For this review, take the finished solid that the model builds, in its own axes (mm). Face numbers are marked on the shaded views. Coordinates: 2 decimals unless noted, no trailing zeros. Write each loop counter-clockwise with the first axis right and the second up, starting at its lowest first coordinate (ties: lowest second). Pieces come first, ordered by that corner, then holes. Notation, with made-up numbers: M 21,37.25 L 49,37.25 A10 cw 49,56.25 Z; hole C 87,52 d7. An arc over 180 degrees is marked long. One line per question, with ' | ' between items.
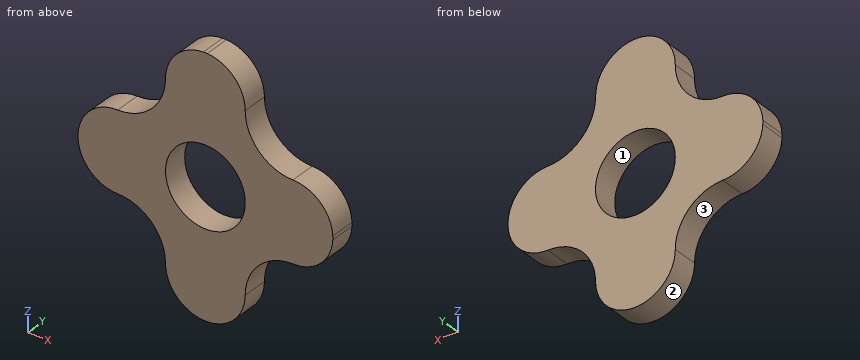
from build123d import *

# Parameters (mm, degrees)
F0_R      = 35.56
F1_DEPTH  = 7.1882
F2_R      = 11.1379
F3_DEPTH  = 7.62
F7_DEPTH  = 7.1882
F9_DEPTH  = 7.1882
F11_DEPTH = 7.1882
F13_DEPTH = 7.1882
F15_DEPTH = 25.4


# Not quite as in the source:
# - a feature of the source that left no trace in its solid (it failed there, or was rolled back) is left out


with BuildPart() as f1:
    # F0 (on Front) → F1 (new body)
    with BuildSketch(Plane.XZ):
        Circle(F0_R)
    extrude(amount=F1_DEPTH)

    # F2 (on face) → F3 (cut)
    with BuildSketch(Plane(origin=(0, 0, 0), x_dir=(-1, 0, 0), z_dir=(0, 1, 0))):
        Circle(F2_R)
    extrude(amount=-F3_DEPTH, mode=Mode.SUBTRACT)

    # F6 (on face) → F7 (join)
    with BuildSketch(Plane.XZ.offset(7.1882)):
        with BuildLine():
            Line((35.56, 11.1379), (33.7707089589, 11.1379))
            ThreePointArc((33.7707089589, 11.1379), (35.1098277593, 5.6403541298), (35.56, 0))
            Line((35.56, 0), (35.56, 11.1379))
        make_face()
        with BuildLine():
            Line((35.56, -11.1125), (35.56, 0))
            ThreePointArc((35.56, 0), (35.1119461572, -5.6271517709), (33.7790755313, -11.1125))
            Line((33.7790755313, -11.1125), (35.56, -11.1125))
        make_face()
    extrude(amount=-F7_DEPTH)

    # F8 (on face) → F9 (join)
    with BuildSketch(Plane.XZ.offset(7.1882)):
        with BuildLine():
            Line((-11.1379, 35.56), (-11.1379, 33.7707089589))
            ThreePointArc((-11.1379, 33.7707089589), (-5.6403540801, 35.1098277673), (1.006e-07, 35.56))
            Line((1.006e-07, 35.56), (-11.1379, 35.56))
        make_face()
        with BuildLine():
            Line((11.1125, 35.56), (1.006e-07, 35.56))
            ThreePointArc((1.006e-07, 35.56), (5.6271518206, 35.1119461492), (11.1125, 33.7790755313))
            Line((11.1125, 33.7790755313), (11.1125, 35.56))
        make_face()
    extrude(amount=-F9_DEPTH)

    # F10 (on face) → F11 (join)
    with BuildSketch(Plane.XZ.offset(7.1882)):
        with BuildLine():
            ThreePointArc((-35.56, 0), (-35.1119461572, 5.627151771), (-33.7790755313, 11.1125))
            Line((-33.7790755313, 11.1125), (-35.56, 11.1125))
            Line((-35.56, 11.1125), (-35.56, 0))
        make_face()
        with BuildLine():
            Line((-35.56, -11.1379), (-33.7707089589, -11.1379))
            ThreePointArc((-33.7707089589, -11.1379), (-35.1098277593, -5.6403541298), (-35.56, 0))
            Line((-35.56, 0), (-35.56, -11.1379))
        make_face()
    extrude(amount=-F11_DEPTH)

    # F12 (on face) → F13 (join)
    with BuildSketch(Plane.XZ.offset(7.1882)):
        with BuildLine():
            ThreePointArc((0, -35.56), (-5.6403541298, -35.1098277593), (-11.1379, -33.7707089589))
            Line((-11.1379, -33.7707089589), (-11.1379, -35.56))
            Line((-11.1379, -35.56), (0, -35.56))
        make_face()
        with BuildLine():
            Line((11.1125, -35.56), (11.1125, -33.7790755313))
            ThreePointArc((11.1125, -33.7790755313), (5.6271517709, -35.1119461572), (0, -35.56))
            Line((0, -35.56), (11.1125, -35.56))
        make_face()
    extrude(amount=-F13_DEPTH)

    # F14 (on face) → F15 (cut)
    with BuildSketch(Plane.XZ.offset(7.1882)):
        with BuildLine():
            ThreePointArc((-11.1379, 24.4221), (-8.0739891454, 32.1147190965), (-0.5444488019, 35.56))
            Line((-0.5444488019, 35.56), (-11.1379, 35.56))
            Line((-11.1379, 35.56), (-11.1379, 33.7707089589))
            ThreePointArc((-11.1379, 33.7707089589), (-25.1541702512, 25.1352604716), (-33.7790755313, 11.1125))
            Line((-33.7790755313, 11.1125), (-35.56, 11.1125))
            Line((-35.56, 11.1125), (-35.56, 0.5190198064))
            ThreePointArc((-35.56, 0.5190198064), (-32.1239164631, 8.03980237), (-24.4475, 11.1125))
            ThreePointArc((-24.4475, 11.1125), (-15.0361915851, 15.0107915851), (-11.1379, 24.4221))
        make_face()
        with BuildLine():
            Line((-0.5444488019, 35.56), (0.5190198064, 35.56))
            ThreePointArc((0.5190198064, 35.56), (-0.0127144977, 35.5727144977), (-0.5444488019, 35.56))
        make_face()
        with BuildLine():
            ThreePointArc((0.5190198064, 35.56), (8.03980237, 32.1239164631), (11.1125, 24.4475))
            ThreePointArc((11.1125, 24.4475), (15.0107915851, 15.0361915851), (24.4221, 11.1379))
            ThreePointArc((24.4221, 11.1379), (32.1147190965, 8.0739891454), (35.56, 0.5444488019))
            Line((35.56, 0.5444488019), (35.56, 11.1379))
            Line((35.56, 11.1379), (33.7707089589, 11.1379))
            ThreePointArc((33.7707089589, 11.1379), (25.1352604716, 25.1541702512), (11.1125, 33.7790755313))
            Line((11.1125, 33.7790755313), (11.1125, 35.56))
            Line((11.1125, 35.56), (0.5190198064, 35.56))
        make_face()
        with BuildLine():
            ThreePointArc((35.56, -0.5190198064), (35.5727144977, 0.0127144977), (35.56, 0.5444488019))
            Line((35.56, 0.5444488019), (35.56, -0.5190198064))
        make_face()
        with BuildLine():
            Line((35.56, -11.1125), (35.56, -0.5190198064))
            ThreePointArc((35.56, -0.5190198064), (32.1239164631, -8.03980237), (24.4475, -11.1125))
            ThreePointArc((24.4475, -11.1125), (15.0182310729, -15.0182310729), (11.1125, -24.4475))
            ThreePointArc((11.1125, -24.4475), (-0.0253855106, -35.5473072489), (-11.1379, -24.4221))
            ThreePointArc((-11.1379, -24.4221), (-15.0287520974, -15.0287520974), (-24.4221, -11.1379))
            ThreePointArc((-24.4221, -11.1379), (-32.1147190965, -8.0739891454), (-35.56, -0.5444488019))
            Line((-35.56, -0.5444488019), (-35.56, -11.1379))
            Line((-35.56, -11.1379), (-33.7707089589, -11.1379))
            ThreePointArc((-33.7707089589, -11.1379), (-25.144717139, -25.144717139), (-11.1379, -33.7707089589))
            Line((-11.1379, -33.7707089589), (-11.1379, -35.56))
            Line((-11.1379, -35.56), (11.1125, -35.56))
            Line((11.1125, -35.56), (11.1125, -33.7790755313))
            ThreePointArc((11.1125, -33.7790755313), (25.144717139, -25.144717139), (33.7790755313, -11.1125))
            Line((33.7790755313, -11.1125), (35.56, -11.1125))
        make_face()
        with BuildLine():
            Line((-35.56, -0.5444488019), (-35.56, 0.5190198064))
            ThreePointArc((-35.56, 0.5190198064), (-35.5727144977, -0.0127144977), (-35.56, -0.5444488019))
        make_face()
    extrude(amount=-F15_DEPTH, mode=Mode.SUBTRACT)


solid = f1.part
1. Take a section at D-D on z = -29. State the section outline as (x, y) points, plus the area to 3 significant figures.
Computed values:
outline: M -10.15,-7.19 L 10.13,-7.19 L 10.13,0 L -10.15,0 Z | area: 146 mm2
2. Clearance check with flat-ended pins moving along their axes: P1, Ø1.5, axis at x = 24.5, y = -6.5, coming from the +Z side; P2, Ø20, axis at x = 0, z = 0, coming from the +Y side. State where each tip first meets the part, or that it passes through.
Computed values:
P1: stops at z = 11.15 | P2: passes through
3. Draft analysis for pull direction X (two halves, no side actions). For the marked faces 1, 2 and 3, state which applies: pulls with the +X half, pulls with the -X half, needs draft (parallel to the pull), parting line crosses it, or undercut.
Computed values:
face 1: undercut | face 2: parting line crosses it | face 3: pulls with the -X half
4. Take a section at C-C on z = -17. State the section outline as (x, y) points, plus the area to 3 significant figures.
Computed values:
outline: M -13.4,-7.19 L 13.39,-7.19 L 13.39,0 L -13.4,0 Z | area: 193 mm2
5. For line 1 along Z through (x, y) = (0, -3.5); line 2 along X through (y, z) = (-5.25, 6.5); line 3 along Z through (x, y) = (3.5, -1), list the stretches that pass through material, from the lowest coordinate up.
Computed values:
line 1: z = -35.55 to -11.14, 11.14 to 35.56 | line 2: x = -33.47 to -9.04, 9.04 to 33.49 | line 3: z = -34.98 to -10.57, 10.57 to 35
6. Take a section at B-B on z = 3. State the section outline as (x, y) points.
Computed values:
outline: M -35.16,-7.19 L -10.73,-7.19 L -10.73,0 L -35.16,0 Z; M 10.73,-7.19 L 35.16,-7.19 L 35.16,0 L 10.73,0 Z
7. Take a section at A-A on y = -3. State the section outline as (x, z) points (1 decimal), plus the area to 3 significant figures.
Computed values:
outline: M -35.6,-0.5 A11.1 ccw -24.4,-11.1 A13.3 cw -11.1,-24.4 A11.1 ccw 11.1,-24.4 A13.3 cw 24.4,-11.1 A11.1 ccw 35.6,-0.5 L 35.6,0.5 A11.1 ccw 24.4,11.1 A13.3 cw 11.1,24.4 A11.1 ccw 0.5,35.6 L -0.5,35.6 A11.1 ccw -11.1,24.4 A13.3 cw -24.4,11.1 A11.1 ccw -35.6,0.5 Z; hole C 0,0 d22.3 | area: 2,220 mm2
